Here's how the part is built. I have some questions about the finished solid (model axes, mm). A direction names the side the tool comes from. Give positions to 0.01 mm unless a question says otherwise; leave off trailing zeros. Write each loop counter-clockwise with the first axis right and the second up, starting at its lowest first coordinate (ties: lowest second). Pieces come first, ordered by that corner, then holes. Notation, with made-up numbers: (16.5, -3) -> (66.5, -3) arc R13 ccw to (66.5, 19) -> close; hole circle Ø6 at (-32.5, 2). An arc over 180 degrees is marked (long way). Use one line per item in the form item = value.
```python
from build123d import *

# Parameters (mm, degrees)
F0_R     = 4.9657
F1_DEPTH = 3.175
F2_R     = 12.7


with BuildPart() as f1:
    # F0 (on Front) → F1 (new body, symmetric)
    with BuildSketch(Plane.XZ):
        Polygon((-55.2147151877, -14.7947383449), (0, 0), (0, 85.4620486929), (-123.7423807387, 52.3053777044), (-102.3768685655, -27.4317992558), align=None)
        with BuildLine():
            ThreePointArc((-53.5360170605, -2.527480351), (-54.5621623786, -5.550406979), (-57.2164993282, -7.3239782266))
            ThreePointArc((-57.2164993282, -7.3239782266), (-63.2982149361, -3.8126980833), (-59.7869347928, 2.2690175246))
            ThreePointArc((-59.7869347928, 2.2690175246), (-55.4787904325, 1.4120743309), (-53.5360170605, -2.527480351))
        make_face(mode=Mode.SUBTRACT)
        with Locations((-90.9608605544, 3.5666267904)):
            Circle(F0_R, mode=Mode.SUBTRACT)
        with BuildLine():
            ThreePointArc((-64.6296483812, 38.8745153783), (-65.6557936993, 35.8515887503), (-68.310130649, 34.0780175027))
            ThreePointArc((-68.310130649, 34.0780175027), (-73.5349030631, 41.8974420064), (-64.6296483812, 38.8745153783))
        make_face(mode=Mode.SUBTRACT)
        with Locations((-102.0544918751, 44.9686225197)):
            Circle(F0_R, mode=Mode.SUBTRACT)
        Polygon((0, 85.4620486929), (0, 0), (102.3768685655, -27.4317992558), (123.7423807387, 52.3053777044), align=None)
        with Locations((58.5017170605, -2.527480351)):
            Circle(F0_R, mode=Mode.SUBTRACT)
        with Locations((90.9608605544, 3.5666267904)):
            Circle(F0_R, mode=Mode.SUBTRACT)
        with Locations((69.5953483812, 38.8745153783)):
            Circle(F0_R, mode=Mode.SUBTRACT)
        with Locations((102.0544918751, 44.9686225197)):
            Circle(F0_R, mode=Mode.SUBTRACT)
    extrude(amount=F1_DEPTH, both=True)

    # F2
    f2_edges = [f1.edges().sort_by_distance(p)[0] for p in [
        (-123.742381, 0, 52.305378),
        (0, 0, 85.462049),
        (0, 0, 0),
        (102.376869, 0, -27.431799),
        (123.742381, 0, 52.305378),
        (-102.376869, 0, -27.431799),
    ]]
    fillet(f2_edges, radius=F2_R)


solid = f1.part
```
Q1. Will these pins go through, and if not, where does the flat tip stop? pin 1 Ø1.5 at (x, y) = (94.5, 1) entering from -Z; pin 2 Ø1 at (x, y) = (-52, 0.5) entering from +Z; pin 3 Ø2 at (x, y) = (11.5, 0.5) entering from +Z.
Result set:
pin_1 = -24.57
pin_2 = 71.66
pin_3 = 82.65
Q2. I want a section at C-C, the plane x = 7.5. Write out the boundary of the cut face in (y, z) (3 decimals).
Result set:
outline = (-3.175, -2.01) -> (3.175, -2.01) -> (3.175, 83.452) -> (-3.175, 83.452) -> close
Q3. Which directions (+Z, -Z, +X, -X, +Y, -Y) give clear straight access to the entire face, cutting with the end or side of a thin tool? Please do faces 1 (the face through (-2, -3.175, 31)), 2 (the face through (46.09, -0.04, -12.35)).
Result set:
face_1 = +Z, -Z, +X, -X, -Y
face_2 = -Z, +Y, -Y
Q4. I want a section at A-A, the plane y = 0. Count the separate pieces of the cut face and the enclosed holes in it, and give its area (3 significant figures).
Result set:
separate_pieces = 1
enclosed_holes = 8
area = 18,600 mm2
Q5. If I drill on line 1 along Z through (x, y) = (-87, 1.25); line 2 along X through (y, z) = (2.25, 48.5); line 3 along Z through (x, y) = (-1, 0.25), over which ranges is the centre line in solid material (lowest first)? Write a range as from..to.
Result set:
line_1 = -23.31..0.57, 6.56..62.15
line_2 = -119.79..-105.55, -98.56..98.56, 105.55..119.79
line_3 = -0.49..84.97
Q6. If we mould it in two halves opening along X, with no side actions, what happens to faces 3 (the face through (-2, 3.175, 31)), 4 (the face through (-0.05, -0.04, -0.45)), 5 (the face through (-0.047, 0.044, 85.014))? For each: +X half, -X half, draft (parallel to the pull), parting line (faces both ways), or undercut.
Result set:
face_3 = draft
face_4 = undercut
face_5 = parting line
Q7. I want a section at B-B, the plane z = 29. Write out the boundary of the cut face in (x, y) (3 decimals), and give its area (3 significant figures).
Result set:
outline = (-117.498, -3.175) -> (117.498, -3.175) -> (117.498, 3.175) -> (-117.498, 3.175) -> close
area = 1,490 mm2
